Here's the drawing with two shaded views (mm, measured from the low corner). I have some questions. A direction names the side the tool comes from. Round coordinates to 2 decimals unless told otherwise and drop trailing zeros. Write each loop counter-clockwise with the first axis right and the second up, starting at its lowest first coordinate (ties: lowest second). Pieces come first, ordered by that corner, then holes.
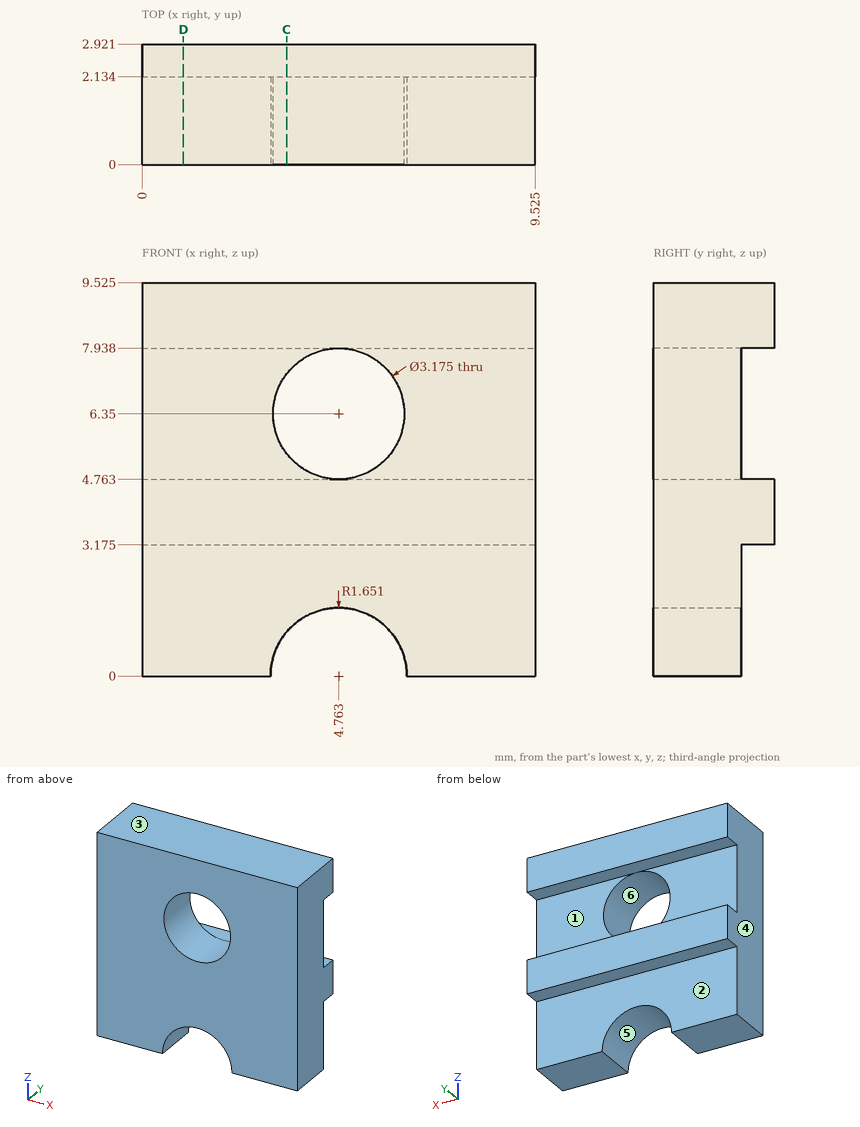
Q1. I'm going to push flat-ended pins straight in: pin 1 Ø1.6 at (x, z) = (7, 1) entering from +Y; pin 2 Ø2.5 at (x, z) = (4.76, 6.35) entering from +Y. Where does each tip first touch, or does it pass through?
Q2. Imagine slicing it at D-D, the plane x = 1. Write out the boundary of the cut face in (y, z) (1 decimal).
Q3. Imagine slicing it at C-C, the plane x = 3.5. Write out the boundary of the cut face in (y, z) (1 decimal).
Q4. On a 3-axis mill with a long thin cutter (end or side, diameter ignored), from which of +Z, -Z, +X, -X, +Y, -Y can I reach the whole of each face in a straight line? I mean the marked faces 1, 2 and 3. Say none if no direction works.
Q5. We'd pull the mould along Z, two halves only. Please class the marked faces 4, 5 and 6: pulls with the +Z half, pulls with the -Z half, needs draft (parallel to the pull), parting line crosses it, or undercut.
Q6. If I drill on L1, parallel to Z at x = 5.5, y = 2.55 (1 decimal); L2, parallel to Y at x = 0.5, z = 2.5; L3, parallel to X at y = 1.4, z = 5.75 (1 decimal), over which ranges is the centre line in solid material (lowest first)?
Results found:
1. pin 1: stops at y = 2.13
1. pin 2: passes through
2. outline: (0, 0) - (2.1, 0) - (2.1, 3.2) - (2.9, 3.2) - (2.9, 4.8) - (2.1, 4.8) - (2.1, 7.9) - (2.9, 7.9) - (2.9, 9.5) - (0, 9.5) - close
3. outline: (0, 1.1) - (2.1, 1.1) - (2.1, 3.2) - (2.9, 3.2) - (2.9, 4.8) - (2.1, 4.8) - (2.1, 5.4) - (0, 5.4) - close; (0, 7.3) - (2.1, 7.3) - (2.1, 7.9) - (2.9, 7.9) - (2.9, 9.5) - (0, 9.5) - close
4. face 1: +X, -X, +Y
4. face 2: -Z, +X, -X, +Y
4. face 3: +Z, +X, -X, +Y, -Y
5. face 4: needs draft
5. face 5: pulls with the -Z half
5. face 6: undercut
6. L1: z = 3.2 to 4.8, 7.9 to 9.5
6. L2: y = 0 to 2.13
6. L3: x = 0 to 3.3, 6.2 to 9.5
